Input: dimensioned drawing with shaded views. Units: mm. Origin: part minimum x, y, z. Give positions to 0.01 mm unless a question says otherwise; leave off trailing zeros. Order: outer loops, then holes, each group sorted by start corner. A loop starts at its lowest first (then second) coordinate and runs counter-clockwise, first axis right, second up.
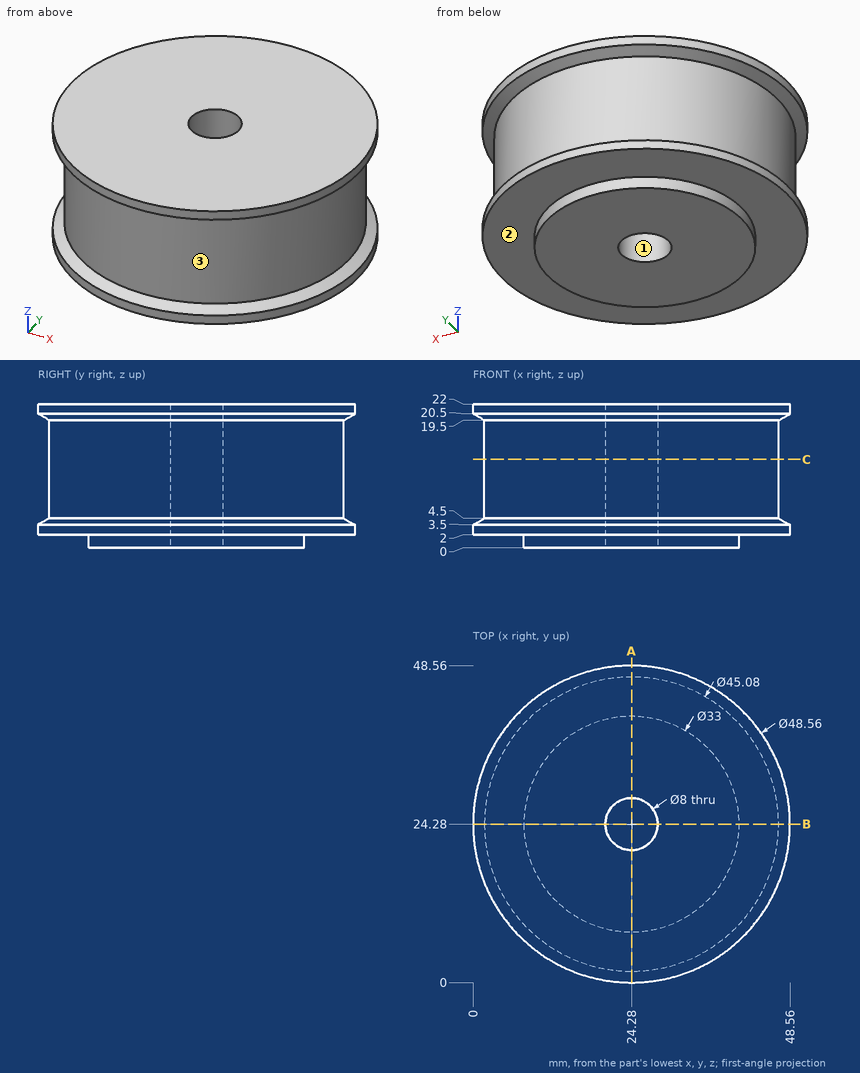
1) Pin query (flat end, axial travel): pin 1 (2 mm diameter, centred on y = 12.5, z = 14, fed in from -X) (3 decimals); pin 2 (3 mm diameter, centred on x = 7.5, z = 8.5, fed in from -Y); pin 3 (6.5 mm diameter, centred on x = 24.28, y = 24.28, fed in from -Z); pin 4 (2 mm diameter, centred on x = 34.5, z = 3, fed in from +Y). Return the tip coordinate at first contact, or that it passes through.
Report:
pin 1: stops at x = 4.485
pin 2: stops at y = 7.71
pin 3: passes through
pin 4: stops at y = 46.74
2) Draft query along Y for the marked faces 1, 2 and 3. Return one class per face: +Y half, -Y half, draft (parallel to the pull), parting line (faces both ways), or undercut.
Report:
face 1: undercut
face 2: draft
face 3: parting line
3) Material intervals for L1, parallel to Y at x = 24.28, z = 5.5; L2, parallel to Z at x = 6.5, y = 25.5; L3, parallel to Y at x = 25.5, z = 13.5, sorted ascending.
Report:
L1: y = 1.74 to 20.28, 28.28 to 46.82
L2: z = 2 to 22
L3: y = 1.77 to 20.47, 28.09 to 46.79
4) Section query C-C, the plane z = 13.5. Return the cut outline in (x, y).
Report:
outline: circle Ø45.08 at (24.28, 24.28); hole circle Ø8 at (24.28, 24.28)
5) Section query A-A, the plane x = 24.28. Return the cut outline in (y, z).
Report:
outline: (0, 2) - (7.78, 2) - (7.78, 0) - (20.28, 0) - (20.28, 22) - (0, 22) - (0, 20.5) - (1.74, 19.5) - (1.74, 4.5) - (0, 3.5) - close; (28.28, 0) - (40.78, 0) - (40.78, 2) - (48.56, 2) - (48.56, 3.5) - (46.82, 4.5) - (46.82, 19.5) - (48.56, 20.5) - (48.56, 22) - (28.28, 22) - close
